Geometry check sheet. Reference: the model listing, model coordinates, mm. Face numbers are marked on the shaded views. A direction names the side the tool comes from. Give positions to 0.01 mm unless a question says otherwise; leave off trailing zeros. Loops run counter-clockwise (first coordinate to the right, second up) from the corner with the lowest first, then second, coordinate; pieces in that order, holes last. Notation, with made-up numbers: (85.5, 75) -> (89.5, 75) arc R30 cw to (89.5, 114) -> close; hole circle Ø7 at (37, 30.25). An arc over 180 degrees is marked (long way). Write each question's results on one line, items separated by ' | '. Start each with the question number.
1) Depth check by flat-ended pin: pin 1 (12 mm diameter, centred on y = 4.5, z = 33, fed in from +X); pin 2 (3 mm diameter, centred on y = -9.5, z = 5, fed in from -X); pin 3 (2.5 mm diameter, centred on x = 2.5, y = 6.5, fed in from +Z). Enter the tip coordinate at first touch or a pass-through.
2) Sectioned sample at D-D on z = 31. Record the cut outline in (x, y).
3) Set-up check for the marked faces 1 and 2: record each of +Z, -Z, +X, -X, +Y, -Y from which the full face is reachable in a straight line by a thin tool's end or side.
4) Scan lines: line 1 (Y direction, x = 1.1, z = 0); line 2 (Y direction, x = 1.35, z = 11); line 3 (Z direction, x = 1.75, y = 2.25). Record each from-to range of solid material in increasing order. Write a range as from..to.
5) Sectioned sample at B-B on z = 0. Record the cut outline in (x, y), then the cut area to 3 significant figures.
6) Sectioned sample at A-A on y = -7.5. Record the cut outline in (x, z).
7) Sectioned sample at C-C on x = 4.35. Record the cut outline in (y, z), then the cut area to 3 significant figures.
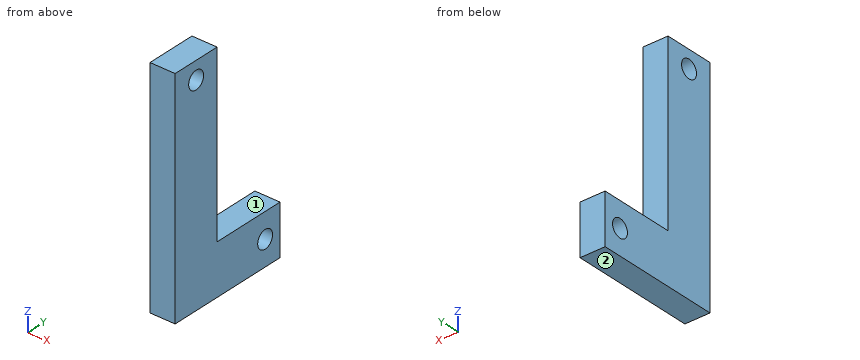
```python
from build123d import *

# Parameters (mm, degrees)
BOSS_EXTRUDE1_DEPTH          = 5
F_5_32_0_14_DIAMETER_HOLE1_D = 3.556


with BuildPart() as part:
    # Sketch1 → Boss-Extrude1 (new body)
    with BuildSketch(Plane(origin=(0, 0, 0), x_dir=(0, 0, -1), z_dir=(1, 0, 0))):
        Polygon((-40, -2.5), (-5, -2.5), (-5, 12.5), (5, 12.5), (5, -2.5), (5, -12.5), (-40, -12.5), align=None)
    extrude(amount=BOSS_EXTRUDE1_DEPTH)

    # 5/32 (0.14) Diameter Hole1 (through all)
    with Locations(Plane(origin=(5, 0, 0), x_dir=(0, 0, -1), z_dir=(1, 0, 0))):
        with Locations((0, 8.957513111), (-36.457513111, -7.5)):
            Hole(F_5_32_0_14_DIAMETER_HOLE1_D / 2)


solid = part.part
```
Result:
1) pin 1: through | pin 2: x = 0 | pin 3: z = 5
2) outline: (0, -12.5) -> (5, -12.5) -> (5, -2.5) -> (0, -2.5) -> close
3) face 1: +Z, +X, -X, +Y | face 2: -Z, +X, -X, +Y, -Y
4) line 1: -12.5..7.18, 10.74..12.5 | line 2: -12.5..-2.5 | line 3: -5..5
5) outline: (0, -12.5) -> (5, -12.5) -> (5, 7.18) -> (0, 7.18) -> close; (0, 10.74) -> (5, 10.74) -> (5, 12.5) -> (0, 12.5) -> close | area: 107 mm^2
6) outline: (0, -5) -> (5, -5) -> (5, 34.68) -> (0, 34.68) -> close; (0, 38.24) -> (5, 38.24) -> (5, 40) -> (0, 40) -> close
7) outline: (-12.5, -5) -> (12.5, -5) -> (12.5, 5) -> (-2.5, 5) -> (-2.5, 40) -> (-12.5, 40) -> close; hole circle Ø3.56 at (-7.5, 36.46); hole circle Ø3.56 at (8.96, 0) | area: 580 mm^2
